The model under review builds one solid part; all positions refer to its coordinate system, in mm. A direction names the side the tool comes from. Round coordinates to 2 decimals unless told otherwise and drop trailing zeros. Write each loop counter-clockwise with the first axis right and the second up, starting at its lowest first coordinate (ties: lowest second). Pieces come first, ordered by that corner, then holes. Notation, with made-up numbers: M 62.5,55.5 L 88.5,55.5 A25 ccw 88.5,83.5 Z; hole C 38,23.5 d11. An arc over 180 degrees is marked long. One line per item, written item: value. Start each with the question number.
1) For P1, Ø12, axis at x = 7, z = -5, coming from the +Y side; P2, Ø1.5, axis at x = 13, z = 3, coming from the -Y side; P3, Ø2, axis at y = -5.5, z = -0.5, coming from the -X side, all flat-tipped, find the tip position at first contact; note any pin that passes through.
2) Take a section at A-A, the plane z = 7.75. Write out the cut boundary in (x, y), and give its area (3 significant figures).
3) Tool access review of faces 1 (the face through (25.84, 49.68, 8.25)), 2 (the face through (25.379, 48.794, -7.743)), 3 (the face through (-52, 46, 1.042)): name each direction out of +Z, -Z, +X, -X, +Y, -Y from which nothing blocks a thin tool from reaching the whole face with its end or side.
4) Mouldability with a two-part tool opening along Y and no side actions: class faces 4 (the face through (-52, 46, -1.042)), 5 (the face through (-39, 43, 1.042)), 6 (the face through (33.45, 64.32, -8.13)) as +Y half, -Y half, draft (parallel to the pull), parting line (faces both ways), or undercut.
5) Take a section at B-B, the plane z = -9. Write out the cut boundary in (x, y), and give its area (3 significant figures).
6) Wall thickness on probe 1 along Z at (x, y) = (64.5, -23); probe 2 along X at (y, z) = (-1.5, -5.25); probe 3 along Y at (x, z) = (0, 0.15): over which ranges is each line inside the solid? List them lowest first.
from build123d import *
from build123d.topology import SkipClean

# Parameters (mm, degrees)
FILLET1_R       = 1
CAGESKE_W       = 2.083334
CAGESKE_H       = 12.5
SIMPLIFIEDSKE_R = 5.208333


with BuildPart() as part:
    # BaseSke → Ball (revolve)
    with BuildSketch(Plane(origin=(0, 0, 0), x_dir=(0, 0, -1), z_dir=(1, 0, 0))):
        with BuildLine():
            Line((0, 68.958333), (0, 58.541667))
            ThreePointArc((0, 58.541667), (-5.208333, 63.75), (0, 68.958333))
        make_face()
    revolve(axis=Axis((0, 68.958333, 0), (0, -1, 0)))

    # InnerRaceSke → InnerRace (revolve)
    with BuildSketch(Plane(origin=(0, 0, 0), x_dir=(0, 0, -1), z_dir=(1, 0, 0)), mode=Mode.PRIVATE) as innerrace_sk:
        with BuildLine():
            Line((3.87931, 60.289708), (3.87931, 55))
            Line((3.87931, 55), (12.5, 55))
            Line((12.5, 55), (12.5, 72.5))
            Line((12.5, 72.5), (3.87931, 72.5))
            Line((3.87931, 72.5), (3.87931, 67.210292))
            ThreePointArc((3.87931, 67.210292), (5.198333, 63.75), (3.87931, 60.289708))
        make_face()
    revolve(innerrace_sk.sketch.rotate(Axis((0, 0, 18.959038), (0, 0, -1)), 90), axis=Axis((0, 0, 18.959038), (0, 0, -1)))

    # OuterRaceSke → OuterRace (revolve)
    with BuildSketch(Plane(origin=(0, 0, 0), x_dir=(0, 0, -1), z_dir=(1, 0, 0)), mode=Mode.PRIVATE) as outerrace_sk:
        with BuildLine():
            Line((-3.87931, 60.289708), (-3.87931, 56))
            Line((-3.87931, 56), (-12.5, 56))
            Line((-12.5, 56), (-12.5, 72.5))
            Line((-12.5, 72.5), (-3.87931, 72.5))
            Line((-3.87931, 72.5), (-3.87931, 67.210292))
            ThreePointArc((-3.87931, 67.210292), (-5.198333, 63.75), (-3.87931, 60.289708))
        make_face()
    revolve(outerrace_sk.sketch.rotate(Axis((0, 0, 27.164344), (0, 0, -1)), 90), axis=Axis((0, 0, 27.164344), (0, 0, -1)))

    # Fillet1
    fillet1_edges = [part.edges().sort_by_distance(p)[0] for p in [
        (-72.5, 0, 12.5),
        (-55, 0, -12.5),
    ]]
    fillet(fillet1_edges, radius=FILLET1_R)

    # CageSke → Cage (revolve)
    with SkipClean():  # the faces are left unmerged after this step: merging them gives an invalid solid
        with BuildSketch(Plane(origin=(0, 0, 0), x_dir=(0, 0, -1), z_dir=(1, 0, 0)), mode=Mode.PRIVATE) as cage_sk:
            with Locations((0, 63.75)):
                Rectangle(CAGESKE_W, CAGESKE_H)
        revolve(cage_sk.sketch.rotate(Axis((0, 0, 23.07703), (0, 0, -1)), 90), axis=Axis((0, 0, 23.07703), (0, 0, -1)))

    # SimplifiedSke → Simplified (revolve)
    with BuildSketch(Plane(origin=(0, 0, 0), x_dir=(0, 0, -1), z_dir=(1, 0, 0)), mode=Mode.PRIVATE) as simplified_sk:
        with Locations((0, 63.75)):
            Circle(SIMPLIFIEDSKE_R)
    revolve(simplified_sk.sketch.rotate(Axis((0, 0, 32.353574), (0, 0, -1)), 90), axis=Axis((0, 0, 32.353574), (0, 0, -1)))


solid = part.part
Checked values:
1. P1: stops at y = 72.49
1. P2: stops at y = -67.23
1. P3: stops at x = -69.86
2. outline: C 0,0 d145; hole C 0,0 d112
2. area: 6,660 mm2
3. face 1: +Z
3. face 2: +Z, -Z
3. face 3: none
4. face 4: draft
4. face 5: undercut
4. face 6: parting line
5. outline: C 0,0 d145; hole C 0,0 d110
5. area: 7,010 mm2
6. probe 1: z = -12.5 to -3.88, -2.18 to 2.18, 3.88 to 12.5
6. probe 2: x = -72.48 to -54.98, 54.98 to 72.48
6. probe 3: y = -70 to -57.5, 57.5 to 70
